```python
from build123d import *

# Parameters (mm, degrees)
SKETCH1_R           = 3
SKETCH1_R_2         = 8
BOSS_EXTRUDE1_DEPTH = 30
BOSS_EXTRUDE2_DEPTH = 120
SKETCH5_W           = 153.62
SKETCH5_H           = 9
SKETCH5_H_2         = 6
BOSS_EXTRUDE3_DEPTH = 150
SKETCH6_W           = 153.62
SKETCH6_H           = 6
BOSS_EXTRUDE4_DEPTH = 150
SKETCH7_W           = 153.62
SKETCH7_H           = 15
SKETCH7_R           = 18.19
BOSS_EXTRUDE5_DEPTH = 10.65
CUT_EXTRUDE1_REACH  = 337.747
SKETCH8_R           = 3
SKETCH8_R_2         = 4


with BuildPart() as part:
    # Sketch1 → Boss-Extrude1 (new body)
    with BuildSketch(Plane.XY):
        with BuildLine():
            Line((-18.19, -47.31), (-18.19, -78.22))
            ThreePointArc((-18.19, -78.22), (0, -96.41), (18.19, -78.22))
            Line((18.19, -78.22), (18.19, -47.31))
            ThreePointArc((18.19, -47.31), (42.5, -23), (66.81, -47.31))
            Line((66.81, -47.31), (66.81, -71.521567483))
            ThreePointArc((66.81, -71.521567483), (74.211608285, -60.407709723), (76.81, -47.31))
            Line((76.81, -47.31), (76.81, 0))
            Line((76.81, 0), (-76.81, 0))
            Line((-76.81, 0), (-76.81, -47.31))
            ThreePointArc((-76.81, -47.31), (-74.211608285, -60.407709723), (-66.81, -71.521567483))
            Line((-66.81, -71.521567483), (-66.81, -47.31))
            ThreePointArc((-66.81, -47.31), (-42.5, -23), (-18.19, -47.31))
        make_face()
        with Locations((0, -83.41)):
            Circle(SKETCH1_R, mode=Mode.SUBTRACT)
        with Locations((0, -37.71)):
            Circle(SKETCH1_R_2, mode=Mode.SUBTRACT)
    extrude(amount=-BOSS_EXTRUDE1_DEPTH)

    # Sketch3 → Boss-Extrude2 (add)
    with BuildSketch(Plane(origin=(0, 0, -30), x_dir=(-1, 0, 0), z_dir=(0, 0, -1))):
        with BuildLine():
            Line((-76.81, 0), (-76.81, -47.31))
            ThreePointArc((-76.81, -47.31), (-74.211608285, -60.407709723), (-66.81, -71.521567483))
            Line((-66.81, -71.521567483), (-66.81, -47.31))
            ThreePointArc((-66.81, -47.31), (-42.5, -23), (-18.19, -47.31))
            Line((-18.19, -47.31), (-18.19, -19.7))
            Line((-18.19, -19.7), (18.19, -19.7))
            Line((18.19, -19.7), (18.19, -47.31))
            ThreePointArc((18.19, -47.31), (42.5, -23), (66.81, -47.31))
            Line((66.81, -47.31), (66.81, -71.521567483))
            ThreePointArc((66.81, -71.521567483), (74.211608285, -60.407709723), (76.81, -47.31))
            Line((76.81, -47.31), (76.81, 0))
            Line((76.81, 0), (-76.81, 0))
        make_face()
    extrude(amount=BOSS_EXTRUDE2_DEPTH)

    # Sketch5 → Boss-Extrude3 (add)
    with BuildSketch(Plane.XY):
        with Locations((0, -4.5)):
            Rectangle(SKETCH5_W, SKETCH5_H)
        with Locations((0, 3)):
            Rectangle(SKETCH5_W, SKETCH5_H_2)
    extrude(amount=BOSS_EXTRUDE3_DEPTH)

    # Sketch6 → Boss-Extrude4 (add)
    with BuildSketch(Plane(origin=(0, 0, 0), x_dir=(-1, 0, 0), z_dir=(0, 0, -1))):
        with Locations((0, 3)):
            Rectangle(SKETCH6_W, SKETCH6_H)
    extrude(amount=BOSS_EXTRUDE4_DEPTH)

    # Sketch7 → Boss-Extrude5 (add)
    with BuildSketch(Plane.XY.offset(150)):
        with BuildLine():
            Line((-76.81, -9), (-14.694324823, -94.13160986))
            ThreePointArc((-14.694324823, -94.13160986), (-5.638542873, -66.115985594), (18.19, -83.41))
            ThreePointArc((18.19, -83.41), (17.294014406, -89.048542873), (14.694324823, -94.13160986))
            Line((14.694324823, -94.13160986), (76.81, -9))
            Line((76.81, -9), (-76.81, -9))
        make_face()
        with Locations((0, -1.5)):
            Rectangle(SKETCH7_W, SKETCH7_H)
        with Locations((0, -83.41)):
            Circle(SKETCH7_R)
    extrude(amount=BOSS_EXTRUDE5_DEPTH)

    # Sketch8 → Cut-Extrude1 (cut, up to next)
    with BuildSketch(Plane.XY.offset(160.65), mode=Mode.PRIVATE) as cut_extrude1_sk1:
        with Locations((0, -83.41)):
            Circle(SKETCH8_R)
    cut_extrude1_tool1 = extrude(cut_extrude1_sk1.sketch, amount=-CUT_EXTRUDE1_REACH, mode=Mode.PRIVATE) & part.part
    # Sketch8 → Cut-Extrude1 (cut, up to next)
    with BuildSketch(Plane.XY.offset(160.65), mode=Mode.PRIVATE) as cut_extrude1_sk2:
        with Locations((0, -37.71)):
            Circle(SKETCH8_R_2)
    cut_extrude1_tool2 = extrude(cut_extrude1_sk2.sketch, amount=-CUT_EXTRUDE1_REACH, mode=Mode.PRIVATE) & part.part
    add(cut_extrude1_tool1.solids().sort_by_distance((0, -83.41, 160.65))[0], mode=Mode.SUBTRACT)
    add(cut_extrude1_tool2.solids().sort_by_distance((0, -37.71, 160.65))[0], mode=Mode.SUBTRACT)


solid = part.part
```
Source: CAD feature listing. Evaluate the final solid. Frame: model axes, mm. A direction names the side the tool comes from. Round coordinates to 2 decimals unless told otherwise and drop trailing zeros. Order: outer loops, then holes, each group sorted by start corner. A loop starts at its lowest first (then second) coordinate and runs counter-clockwise, first axis right, second up. Notation, with made-up numbers: (76, 86.5) -> (95, 86.5) arc R23 cw to (95, 108.5) -> close; hole circle Ø10 at (64, -5). An arc over 180 degrees is marked (long way). Use CSV: the item, a comma, the result in double quotes.
(1) Access query for faces 4 (the face through (-0.4, -96.406, -14.79)), 5 (the face through (-1.041, -29.778, -14.79)), 6 (the face through (66.81, -60, -74)). Directions: +Z, -Z, +X, -X, +Y, -Y. A direction counts if a zero-diameter tool reaches every point of the face in a straight line with its end or side. Return the directions, or none.
Report:
face 4,"-Z, -Y"
face 5,"-Z"
face 6,"+Z, -Z, -Y"
(2) First-contact query: pin 1 Ø24 at (y, z) = (-63.5, -16.5) entering from +X; pin 2 Ø7.5 at (y, z) = (-64, -104) entering from -X; pin 3 Ø6 at (x, y) = (-39, -64.5) entering from -Z. Flat tips, straight axial feed; report the tip coordinate or a pass-through.
Report:
pin 1,"x = 76.55"
pin 2,"x = -74.28"
pin 3,"z = 150"
(3) Section C-C on y = -67.5. Return the cut outline in (x, z).
Report:
outline,"(-70.24, -150) -> (-66.81, -150) -> (-66.81, 0) -> (-70.24, 0) -> close; (-34.13, 150) -> (34.13, 150) -> (34.13, 160.65) -> (-34.13, 160.65) -> close; (-18.19, -30) -> (18.19, -30) -> (18.19, 0) -> (-18.19, 0) -> close; (66.81, -150) -> (70.24, -150) -> (70.24, 0) -> (66.81, 0) -> close"
(4) Ray query, L1, parallel to Y at x = 0, z = 157.25; L2, parallel to Z at x = -56.5, y = -18; L3, parallel to Y at x = 0, z = -20. Return the intervals inside material, ascending.
Report:
L1,"-101.6 to -86.41, -80.41 to -41.71, -33.71 to 6"
L2,"-150 to 0, 150 to 160.65"
L3,"-96.41 to -86.41, -80.41 to -45.71, -29.71 to 6"
(5) Section D-D on y = -37.71. Return the cut outline in (x, z), and give its area (3 significant figures).
Report:
outline,"(-76.81, -150) -> (-64.83, -150) -> (-64.83, 0) -> (-76.81, 0) -> close; (-55.86, 150) -> (-4, 150) -> (-4, 160.65) -> (-55.86, 160.65) -> close; (-20.17, -150) -> (-18.19, -150) -> (-18.19, -30) -> (-8, -30) -> (-8, 0) -> (-20.17, 0) -> close; (4, 150) -> (55.86, 150) -> (55.86, 160.65) -> (4, 160.65) -> close; (8, -30) -> (18.19, -30) -> (18.19, -150) -> (20.17, -150) -> (20.17, 0) -> (8, 0) -> close; (64.83, -150) -> (76.81, -150) -> (76.81, 0) -> (64.83, 0) -> close"
area,"5,900 mm^2"
(6) Section B-B on z = -41.5. Return the cut outline in (x, y).
Report:
outline,"(-76.81, -47.31) arc R34.31 ccw to (-66.81, -71.52) -> (-66.81, -47.31) arc R24.31 cw to (-18.19, -47.31) -> (-18.19, -19.7) -> (18.19, -19.7) -> (18.19, -47.31) arc R24.31 cw to (66.81, -47.31) -> (66.81, -71.52) arc R34.31 ccw to (76.81, -47.31) -> (76.81, 6) -> (-76.81, 6) -> close"
(7) Pull-direction query (Z, two-part tool) for faces 1 (the face through (-1, -23, 160.65)), 2 (the face through (-1, -9, 74)), 3 (the face through (18.19, -34, -89)); classes: +Z half, -Z half, draft (parallel to the pull), parting line (faces both ways), or undercut.
Report:
face 1,"+Z half"
face 2,"undercut"
face 3,"draft"
(8) Section A-A on x = 0. Return the cut outline in (y, z).
Report:
outline,"(-101.6, 150) -> (-86.41, 150) -> (-86.41, 160.65) -> (-101.6, 160.65) -> close; (-96.41, -30) -> (-86.41, -30) -> (-86.41, 0) -> (-96.41, 0) -> close; (-80.41, -30) -> (-45.71, -30) -> (-45.71, 0) -> (-80.41, 0) -> close; (-80.41, 150) -> (-41.71, 150) -> (-41.71, 160.65) -> (-80.41, 160.65) -> close; (-33.71, 150) -> (-9, 150) -> (-9, 0) -> (-29.71, 0) -> (-29.71, -30) -> (-19.7, -30) -> (-19.7, -150) -> (6, -150) -> (6, 160.65) -> (-33.71, 160.65) -> close"
